Autodesk Inventor part; units mm, degrees
ref_plane "YZ Plane" through (0, 0, 0) normal (1, 0, 0) x (0, 1, 0)
ref_plane "XZ Plane" through (0, 0, 0) normal (0, 1, 0) x (-1, 0, 0)
ref_plane "XY Plane" through (0, 0, 0) normal (0, 0, 1) x (1, 0, 0)
sketch "Sketch1" plane through (0, 0, 0) normal (0, 0, 1) x (1, 0, 0)
  line L0 (-2.7678, 3.3517) -> (22.6322, 3.3517)
  line L1 (22.6322, 3.3517) -> (22.6322, -47.4483)
  line L2 (22.6322, -47.4483) -> (-2.7678, -47.4483)
  line L3 (-2.7678, -47.4483) -> (-2.7678, 3.3517)
  line L4 (19.5061, 0.2256) -> (0.3583, 0.2256)
  line L5 (0.3583, 0.2256) -> (0.3583, -44.3222)
  line L6 (0.3583, -44.3222) -> (19.5061, -44.3222)
  line L7 (19.5061, -44.3222) -> (19.5061, 0.2256)
  point P0 (0, 0)
  dimension "d0" = 25.4
  dimension "d1" = 50.8
extrude "Extrusion1" add sketch "Sketch1" along normal blind 1016
sketch "Sketch2" plane through (-2.7678, 3.3517, 0) normal (0, 1, 0) x (1, 0, 0)
  point P0 (2.7678, 0)
sketch "Sketch3" plane through (22.6322, -47.4483, 0) normal (1, 0, 0) x (0, 0, -1)
  line L0 (0, 0) -> (-1016, 0)
  line L1 (0, 50.8) -> (-114.3, 50.8)
  line L2 (-114.3, 50.8) -> (-114.3, 0)
  line L3 (-114.3, 0) -> (0, 0)
  line L4 (0, 0) -> (0, 50.8)
  line L5 (-1016, 50.8) -> (-901.7, 50.8)
  line L6 (-901.7, 50.8) -> (-901.7, 0)
  line L7 (-901.7, 0) -> (-1016, 0)
  line L8 (-1016, 0) -> (-1016, 50.8)
  point P0 (0, 47.4483)
  point P1 (-114.3, 25.4)
  point P2 (-901.7, 25.4)
  dimension "d4" = 114.3
  dimension "d5" = 114.3
hole "Hole1" at (22.6322, -22.0483, 901.7) at (22.6322, -22.0483, 114.3) direction (-1, 0, 0) diameter 9.525 end through all
properties part number "40in 2x1 boxbeam"
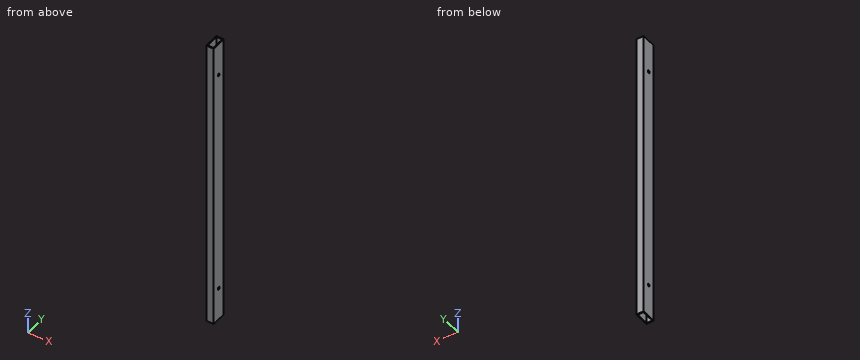
Work out the finished part from the listing and answer in its coordinate system (mm). Round coordinates to 2 decimals unless told otherwise and drop trailing zeros. Loops run counter-clockwise (first coordinate to the right, second up) from the corner with the lowest first, then second, coordinate; pieces in that order, holes last. Notation, with made-up numbers: (39, -15) -> (57, -15) arc R29 cw to (57, 10) -> close; hole circle Ø2 at (82, -0.75). An arc over 180 degrees is marked (long way). Use one line per item in the form item = value.
(1) Straight lines are drawn through the part: line 1 (X direction, y = -18.5, z = 257.5); line 2 (Y direction, x = 5.75, z = 772); line 3 (Z direction, x = 20.25, y = -19.5). For each, find the intervals that lie inside material, in ascending order.
Answer list:
line_1 = -2.77 to 0.36, 19.51 to 22.63
line_2 = -47.45 to -44.32, 0.23 to 3.35
line_3 = 0 to 110.28, 118.32 to 897.68, 905.72 to 1016
(2) Find section C-C on z = 949.5. Give the vertices of the cut face in (x, y).
Answer list:
outline = (-2.77, -47.45) -> (22.63, -47.45) -> (22.63, 3.35) -> (-2.77, 3.35) -> close; hole (0.36, -44.32) -> (19.51, -44.32) -> (19.51, 0.23) -> (0.36, 0.23) -> close
(3) Find section B-B on y = -35.5. Give the vertices of the cut face in (x, z).
Answer list:
outline = (-2.77, 0) -> (0.36, 0) -> (0.36, 1016) -> (-2.77, 1016) -> close; (19.51, 0) -> (22.63, 0) -> (22.63, 1016) -> (19.51, 1016) -> close
(4) A flat-ended cylindrical pin translates along its axis: P1, Ø5.5, axis at y = -22.05, z = 901.7, coming from the -X side. Find the tip coordinate at first contact, or state that the pin passes through.
Answer list:
P1 = through
(5) Find section A-A on x = 5.25. Give the vertices of the cut face in (y, z), then the cut area to 3 significant figures.
Answer list:
outline = (-47.45, 0) -> (-44.32, 0) -> (-44.32, 1016) -> (-47.45, 1016) -> close; (0.23, 0) -> (3.35, 0) -> (3.35, 1016) -> (0.23, 1016) -> close
area = 6,350 mm2
